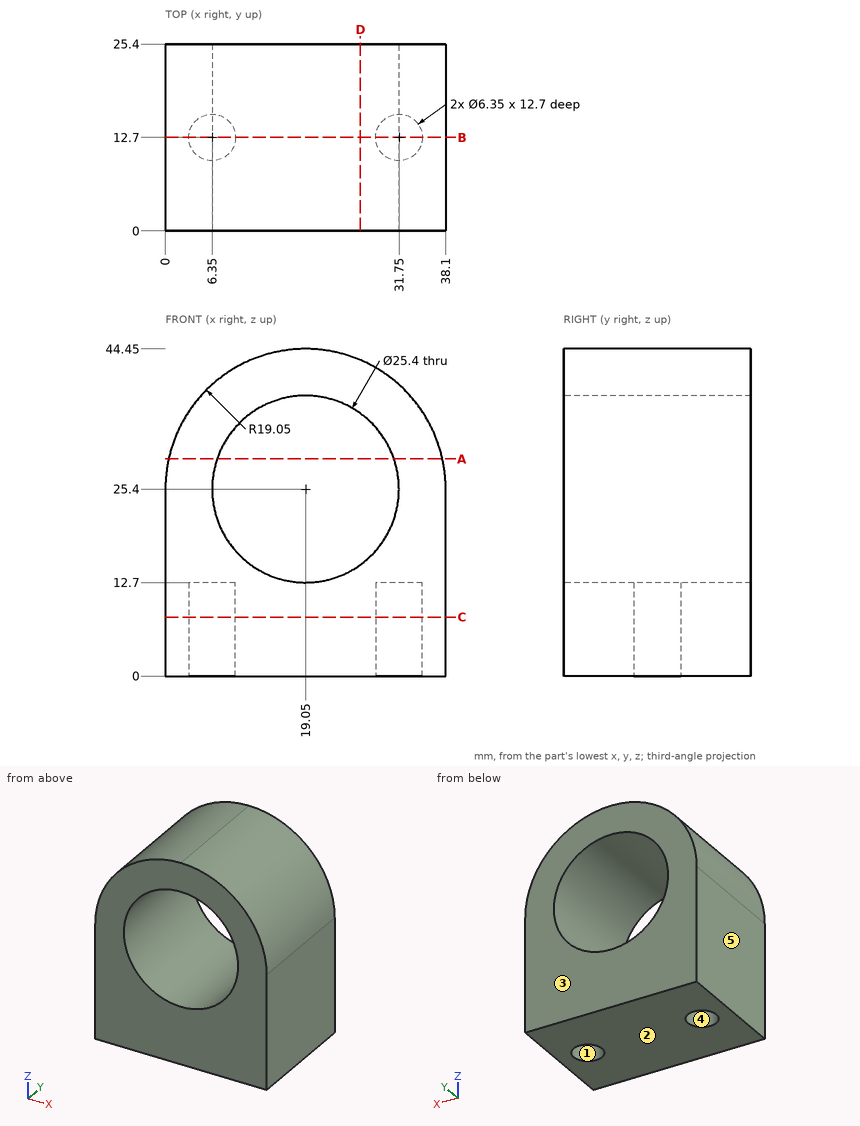
Verification items for this drawing (mm, ordinates from the low corner). A direction names the side the tool comes from. Give positions to 0.01 mm unless a question says otherwise; leave off trailing zeros. Loops run counter-clockwise (first coordinate to the right, second up) from the corner with the lowest first, then second, coordinate; pieces in that order, holes last. Notation, with made-up numbers: M 6.5,-10 L 17.5,-10 A17 cw 17.5,21 Z; hole C -3.5,-32 d4. An arc over 180 degrees is marked long. Return JSON: item names as keys, results as strings. Group by question number.
1. Go/stop test with flat-tipped pins: pin 1 (12 mm diameter, centred on x = 32, y = 17, fed in from +Z); pin 2 (4 mm diameter, centred on x = 31.75, y = 12.7, fed in from -Z); pin 3 (8 mm diameter, centred on x = 28, y = 6.5, fed in from +Z). Record where each tip stops, or that it passes through.
2. Cross-section at B-B on y = 12.7. Record the boundary of the cut face in (x, z) (3 decimals), plus the area to 3 significant figures.
3. Cross-section at A-A on z = 29.5. Record the boundary of the cut face in (x, y), plus the area to 3 significant figures.
4. Thickness scan on L1, parallel to Y at x = 31.75, z = 3.5 (3 decimals); L2, parallel to X at y = 12.7, z = 5.5 (3 decimals); L3, parallel to X at y = 14, z = 9. Record the ranges inside material, lowest first.
5. Tool access check on the marked faces 4 and 5. Record the directions out of +Z, -Z, +X, -X, +Y, -Y that give a thin tool (end or side, any length) a straight path to the whole face; none if there is none.
6. Cross-section at C-C on z = 8. Record the boundary of the cut face in (x, y) (3 decimals), plus the area to 3 significant figures.
7. Cross-section at D-D on x = 26.5. Record the boundary of the cut face in (y, z).
8. Mould release check, pull along Y, two halves, no side actions. Record for the marked faces 1, 2 and 3: released by +Y, released by -Y, zero draft, split by the parting line, or undercut.
Return value:
{
 "1": {"pin 1": "z = 43.14", "pin 2": "z = 12.7", "pin 3": "z = 43.8"},
 "2": {"outline": "M 0,0 L 3.175,0 L 3.175,12.7 L 9.525,12.7 L 9.525,0 L 28.575,0 L 28.575,12.7 L 34.925,12.7 L 34.925,0 L 38.1,0 L 38.1,25.4 A19.05 ccw 19.05,44.45 A19.05 ccw 0,25.4 Z; hole C 19.05,25.4 d25.4", "area": "870 mm^2"},
 "3": {"outline": "M 0.45,0 L 7.03,0 L 7.03,25.4 L 0.45,25.4 Z; M 31.07,0 L 37.65,0 L 37.65,25.4 L 31.07,25.4 Z", "area": "334 mm^2"},
 "4": {"L1": "0 to 9.525, 15.875 to 25.4", "L2": "0 to 3.175, 9.525 to 28.575, 34.925 to 38.1", "L3": "0 to 3.45, 9.25 to 28.85, 34.65 to 38.1"},
 "5": {"face 4": "-Z", "face 5": "+Z, -Z, -X, +Y, -Y"},
 "6": {"outline": "M 0,0 L 38.1,0 L 38.1,25.4 L 0,25.4 Z; hole C 6.35,12.7 d6.35; hole C 31.75,12.7 d6.35", "area": "904 mm^2"},
 "7": {"outline": "M 0,0 L 25.4,0 L 25.4,15.11 L 0,15.11 Z; M 0,35.69 L 25.4,35.69 L 25.4,42.93 L 0,42.93 Z"},
 "8": {"face 1": "undercut", "face 2": "zero draft", "face 3": "released by +Y"}
}
